Check sheet for the modelled part. Datum: model origin and axes. Units: mm. Give positions to 0.01 mm unless a question says otherwise; leave off trailing zeros. Loops run counter-clockwise (first coordinate to the right, second up) from the corner with the lowest first, then second, coordinate; pieces in that order, holes last.
```python
from build123d import *

# Parameters (mm, degrees)
SKETCH_2_W               = 3
SKETCH_2_H               = 32
EXTRUDE_1_DEPTH          = 3
EXTRUDE_2_DEPTH          = 3
EXTRUDE_3_DEPTH          = 3
CUT_EXTRUDE_1_DEPTH      = 64.046222373
CUT_EXTRUDE_1_DEPTH_BACK = 3
SKETCH_6_R               = 0.6
CUT_EXTRUDE_2_DEPTH      = 64.046222373


with BuildPart() as part:
    # 草图2 → 凸台-拉伸1 (new body)
    with BuildSketch(Plane(origin=(0, 0, 0), x_dir=(1, 0, 0), z_dir=(0, 1, 0))):
        with Locations((0, -16)):
            Rectangle(SKETCH_2_W, SKETCH_2_H)
    extrude(amount=EXTRUDE_1_DEPTH)

    # 草图3 → 凸台-拉伸2 (add)
    with BuildSketch(Plane(origin=(1.5, 0, 0), x_dir=(0, 0, -1), z_dir=(1, 0, 0))):
        with BuildLine():
            ThreePointArc((-37.829111907, -20.328529058), (-42.573878655, -7.967989086), (-32, 0))
            Line((-32, 0), (-23.339745962, 0))
            ThreePointArc((-23.339745962, 0), (-43.453167914, -2.948606038), (-39.418869699, -22.872673346))
            Line((-39.418869699, -22.872673346), (-7.193042045, -43.009605387))
            Line((-7.193042045, -43.009605387), (-5.603284253, -40.465461099))
            Line((-5.603284253, -40.465461099), (-37.829111907, -20.328529058))
        make_face()
    extrude(amount=-EXTRUDE_2_DEPTH)

    # 草图4 → 凸台-拉伸3 (add)
    with BuildSketch(Plane(origin=(1.5, 0, 0), x_dir=(0, 0, -1), z_dir=(1, 0, 0))):
        with BuildLine():
            Line((-6.657393053, -39.806780816), (0, 0))
            Line((0, 0), (-32, 0))
            ThreePointArc((-32, 0), (-42.573878655, -7.967989086), (-37.829111907, -20.328529058))
            Line((-37.829111907, -20.328529058), (-6.657393053, -39.806780816))
        make_face()
    extrude(amount=-EXTRUDE_3_DEPTH)

    # 草图5 → 切除-拉伸1 (cut, two sides: drawn at the far end of the back side and taken through both)
    with BuildSketch(Plane(origin=(1.5, 0, 0), x_dir=(0, 0, -1), z_dir=(1, 0, 0)).offset(-CUT_EXTRUDE_1_DEPTH_BACK)):
        Polygon((-6.657393053, -39.806780816), (-7.193042045, -43.009605387), (-5.603284253, -40.465461099), align=None)
    extrude(amount=CUT_EXTRUDE_1_DEPTH + CUT_EXTRUDE_1_DEPTH_BACK, mode=Mode.SUBTRACT)

    # 草图6 → 切除-拉伸2 (cut, through all)
    with BuildSketch(Plane(origin=(1.5, 0, 0), x_dir=(0, 0, -1), z_dir=(1, 0, 0))):
        with Locations((-10, 1.5)):
            Circle(SKETCH_6_R)
        with Locations((-44.015771199, -7.554533052)):
            Circle(SKETCH_6_R)
        with Locations((-23.359125072, -31.139147958)):
            Circle(SKETCH_6_R)
    extrude(amount=-CUT_EXTRUDE_2_DEPTH, mode=Mode.SUBTRACT)


solid = part.part
```
(1) Section check A-A on z = 10. Record the boundary of the cut face in (x, y).
(2) Release check for a two-part mould opening along Z. For faces 1 (the face through (0, 1.5, 10.6)), 2 (the face through (0.02, -32.8, 23.53)), 3 (the face through (0, 3, 16)), 4 (the face through (0, 1, 0)) record: pulls with the +Z half, pulls with the -Z half, needs draft (parallel to the pull), parting line crosses it, or undercut.
(3) Section check D-D on y = -24. Record the boundary of the cut face in (x, z).
(4) Material ranges on line 1 (Y direction, x = 0.15, z = 10); line 2 (Z direction, x = -0.75, y = -6.5); line 3 (Y direction, x = -0.8, z = 40.5), recorded low to high.
(5) Section check C-C on x = 0.4. Record the boundary of the cut face in (y, z).
(6) Section check B-B on y = 1.5. Record the boundary of the cut face in (x, z).
(7) Gauge pin test, flat ends, axial feed: pin 1 Ø1 at (x, y) = (1, -26) entering from +Z; pin 2 Ø1.4 at (y, z) = (-31.14, 23.36) entering from -X; pin 3 Ø1.5 at (x, z) = (1, 21.5) entering from -Y. Record the tip position at first contact, or that the pin passes through.
Computed values:
1. outline: (-1.5, -41.26) - (1.5, -41.26) - (1.5, 0.9) - (-1.5, 0.9) - close; (-1.5, 2.1) - (1.5, 2.1) - (1.5, 3) - (-1.5, 3) - close
2. face 1: undercut
2. face 2: pulls with the +Z half
2. face 3: needs draft
2. face 4: pulls with the -Z half
3. outline: (-1.5, 4.01) - (1.5, 4.01) - (1.5, 37.61) - (-1.5, 37.61) - close
4. line 1: y = -41.26 to 0.9, 2.1 to 3
4. line 2: z = 1.09 to 45.26
4. line 3: y = -22.12 to 0.12
5. outline: (-43.01, 7.19) - (0, 0) - (3, 0) - (3, 32) arc R14 ccw to (-22.87, 39.42) - close; hole circle Ø1.2 at (-31.14, 23.36); hole circle Ø1.2 at (-7.55, 44.02); hole circle Ø1.2 at (1.5, 10)
6. outline: (-1.5, 0) - (1.5, 0) - (1.5, 9.4) - (-1.5, 9.4) - close; (-1.5, 10.6) - (1.5, 10.6) - (1.5, 38.3) - (-1.5, 38.3) - close
7. pin 1: stops at z = 35.21
7. pin 2: stops at x = -1.5
7. pin 3: stops at y = -34.54
